Geometry: see drawing. Coordinates: mm, zero at the bounding-box minimum. A direction names the side the tool comes from. Round coordinates to 2 decimals unless told otherwise and drop trailing zeros. Order: outer loops, then holes, each group sorted by start corner. A loop starts at its lowest first (then second) coordinate and runs counter-clockwise, first axis right, second up. Notation, with made-up numbers: (18, -8) -> (35, -8) arc R24 cw to (35, 13) -> close; hole circle Ø10 at (66.5, 23.25). An arc over 180 degrees is marked (long way). One line per item, written item: value. Start each with the question number.
1) Section A-A (x = 14.5). Return the cut outline in (y, z).
2) Section D-D (x = 8.5). Return the cut outline in (y, z).
3) Section C-C (z = 9). Return the cut outline in (x, y).
4) Ray query, L1, parallel to Z at x = 21.5, y = 39.5; L2, parallel to X at y = 2.5, z = 9; L3, parallel to X at y = 41.5, z = 13. Return the intervals inside material, ascending.
5) Pin query (flat end, axial travel): P1, Ø3, axis at x = 20, z = 2.5, coming from the -Y side; P2, Ø0.9, axis at x = 8.5, z = 9, coming from the -Y side; P3, Ø0.9, axis at y = 41, z = 11, coming from the +X side. Return the tip coordinate at first contact, or that it passes through.
6) Section B-B (y = 40). Return the cut outline in (x, z).
7) Reachability of the marked faces 1 and 2 from +Z, -Z, +X, -X, +Y, -Y: full face, straight path, thin tool, end or side. Return the list, or none.
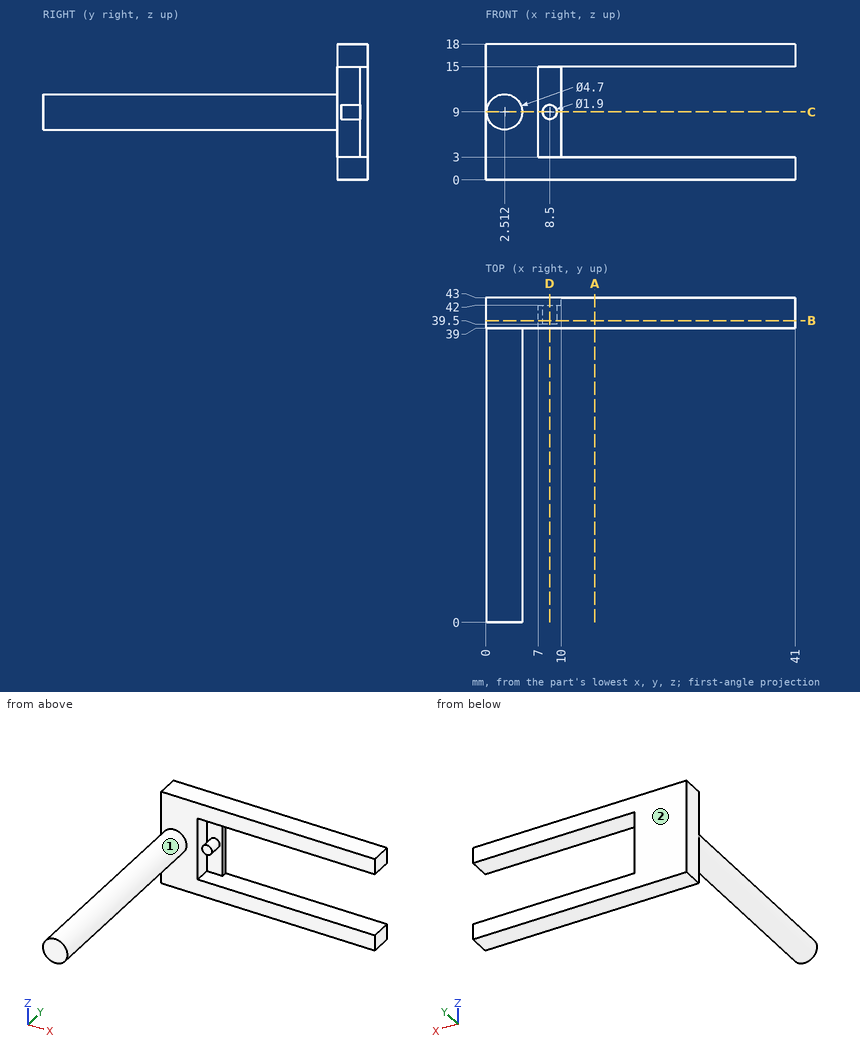
Findings:
1. outline: (39, 0) -> (43, 0) -> (43, 3) -> (39, 3) -> close; (39, 15) -> (43, 15) -> (43, 18) -> (39, 18) -> close
2. outline: (39, 0) -> (43, 0) -> (43, 18) -> (39, 18) -> (39, 15) -> (42, 15) -> (42, 9.95) -> (39.5, 9.95) -> (39.5, 8.05) -> (42, 8.05) -> (42, 3) -> (39, 3) -> close
3. outline: (0, 39) -> (0.16, 39) -> (0.16, 0) -> (4.86, 0) -> (4.86, 39) -> (7, 39) -> (7, 42) -> (7.55, 42) -> (7.55, 39.5) -> (9.45, 39.5) -> (9.45, 42) -> (10, 42) -> (10, 43) -> (0, 43) -> close
4. L1: 0 to 3, 15 to 18
4. L2: 0.16 to 4.86
4. L3: 0 to 7
5. P1: y = 39
5. P2: y = 39.5
5. P3: x = 7
6. outline: (0, 0) -> (41, 0) -> (41, 3) -> (7, 3) -> (7, 15) -> (41, 15) -> (41, 18) -> (0, 18) -> close; circle Ø1.9 at (8.5, 9)
7. face 1: -Y
7. face 2: +Z, -Z, +X, -X, +Y
